Part model, mm, in its own coordinate system. A direction names the side the tool comes from. Give positions to 0.01 mm unless a question says otherwise; leave off trailing zeros. Write each loop counter-clockwise with the first axis right and the second up, starting at its lowest first coordinate (ties: lowest second). Pieces come first, ordered by that corner, then holes. Notation, with made-up numbers: M 27.5,27.25 L 54.5,27.25 A26 cw 54.5,62.25 Z; hole C -21.75,64 d1. An arc over 180 degrees is marked long. Answer as CSV lines item,"result". Start each with the question number.
1) Wall check: line 1 along X through (y, z) = (9.5, -1); line 2 along X through (y, z) = (20, 11.5); line 3 along Z through (x, y) = (13, 44). Give the ranges that are in metal, low to high. Write a range as from..to.
2) Slice it at A-A, the plane z = 0. Give the cut face in (x, y).
3) Slice it at D-D, the plane x = -25.5. Give the cut face in (y, z), plus the area to 3 significant figures.
4) Pin check, flat tips, straight feed: pin 1 Ø4 at (x, y) = (50, 12.5) entering from +Z; pin 2 Ø10 at (x, z) = (-51.5, -51) entering from +Y; pin 3 Ø2 at (y, z) = (23, -31.5) entering from -X; pin 4 Ø4 at (x, y) = (0, 38.1) entering from -Z. Stop position of each tip, or through.
5) Mould opens along Y. For faces 4 (the flat face through (-11.94, 27.94, -75.43)), 5 (the cylindrical face through (2.93, 36.88, -18)), 6 (the cylindrical face through (-45.395, 15.062, 62.776)) say: pulls with the +Y half, pulls with the -Y half, needs draft (parallel to the pull), parting line crosses it, or undercut.
6) Slice it at B-B, the plane x = 0. Give the number of separate pieces and of enclosed holes in the cut face, plus the area to 3 significant figures.
7) Tool access for faces 1 (the flat face through (-62, 27.94, -45)), 2 (the flat face through (-63.33, 41.41, -37.69)), 3 (the flat face through (37.69, 41.41, -63.33)): list every direction of +Z, -Z, +X, -X, +Y, -Y with a clear straight run to the whole face (end or side of a thin tool).
```python
from build123d import *

# Parameters (mm, degrees)
SKETCH2_R           = 76.2
BOSS_EXTRUDE1_DEPTH = 50.8
SKETCH3_R           = 71.12
SKETCH3_R_2         = 19.05
CUT_EXTRUDE1_DEPTH  = 44.45
SKETCH4_R           = 17.272
CUT_EXTRUDE2_DEPTH  = 120.1365603
CUT_EXTRUDE3_DEPTH  = 19.05
CIRPATTERN1_COUNT   = 8
SKETCH6_R           = 3.175
CUT_EXTRUDE4_DEPTH  = 25.4
WRAP1_START         = 2.54
WRAP1_DEPTH         = 25.4
CIRPATTERN2_COUNT   = 8


# Read off the part's stored shape, not the designer's step: Wrap1
with BuildPart() as part:
    # Sketch2 → Boss-Extrude1 (new body)
    with BuildSketch(Plane(origin=(0, 0, 0), x_dir=(1, 0, 0), z_dir=(0, 1, 0))):
        with Locations(Location((0, 0, 0), (0, 0, 270))):
            Circle(SKETCH2_R)
    extrude(amount=BOSS_EXTRUDE1_DEPTH)

    # Sketch3 → Cut-Extrude1 (cut)
    with BuildSketch(Plane(origin=(0, 50.8, 0), x_dir=(1, 0, 0), z_dir=(0, 1, 0))):
        with Locations(Location((0, 0, 0), (0, 0, 270))):
            Circle(SKETCH3_R)
        with Locations(Location((0, 0, 0), (0, 0, 270))):
            Circle(SKETCH3_R_2, mode=Mode.SUBTRACT)
    extrude(amount=-CUT_EXTRUDE1_DEPTH, mode=Mode.SUBTRACT)

    # Sketch4 → Cut-Extrude2 (cut, through all)
    with BuildSketch(Plane(origin=(0, 50.8, 0), x_dir=(1, 0, 0), z_dir=(0, 1, 0))):
        with Locations(Location((0, 0, 0), (0, 0, 270))):
            Circle(SKETCH4_R)
    extrude(amount=-CUT_EXTRUDE2_DEPTH, mode=Mode.SUBTRACT)

    # Sketch5 → Cut-Extrude3 (cut)
    with BuildSketch(Plane(origin=(0, 50.8, 0), x_dir=(1, 0, 0), z_dir=(0, 1, 0))):
        with BuildLine():
            Line((-44.991655358, 55.079990451), (-48.205345027, 59.014275484))
            ThreePointArc((-48.205345027, 59.014275484), (-57.719695429, 49.748133227), (-65.480674483, 38.970774553))
            Line((-65.480674483, 38.970774553), (-61.115296184, 36.372722916))
            ThreePointArc((-61.115296184, 36.372722916), (-53.871715734, 46.431591012), (-44.991655358, 55.079990451))
        make_face()
    cut_extrude3 = extrude(amount=-CUT_EXTRUDE3_DEPTH, mode=Mode.SUBTRACT)

    # CirPattern1: Cut-Extrude3 ×8 about axis
    cirpattern1_axis = Axis((0, 0, 0), (0, 1, 0))
    for i in range(1, CIRPATTERN1_COUNT):
        add(cut_extrude3.rotate(cirpattern1_axis, i * 360 / CIRPATTERN1_COUNT), mode=Mode.SUBTRACT)

    # Sketch6 → Cut-Extrude4 (cut, symmetric)
    with BuildSketch(Plane.XY):
        with Locations((0, 38.1)):
            Circle(SKETCH6_R)
    extrude(amount=CUT_EXTRUDE4_DEPTH, both=True, mode=Mode.SUBTRACT)

    # Wrap1 outline → Wrap1 (add)
    with BuildSketch(Plane(origin=(0, 0, 0), x_dir=(1, 0, 0), z_dir=(0, 1, 0)).offset(WRAP1_START)):
        with BuildLine():
            ThreePointArc((75.761080539, -16.182075751), (76.423312697, 12.691657751), (66.463869373, 39.801444294))
            Line((66.463869373, 39.801444294), (65.374297744, 39.148961601))
            ThreePointArc((65.374297744, 39.148961601), (75.170471505, 12.483597787), (74.519095612, -15.916795821))
            Line((74.519095612, -15.916795821), (75.761080539, -16.182075751))
        make_face()
    wrap1 = extrude(amount=WRAP1_DEPTH)

    # CirPattern2: Wrap1 ×8 about axis
    cirpattern2_axis = Axis((0, 0, 0), (0, 1, 0))
    for i in range(1, CIRPATTERN2_COUNT):
        add(wrap1.rotate(cirpattern2_axis, i * 360 / CIRPATTERN2_COUNT))


solid = part.part
```
Found:
1,line 1,"-77.46..-71.11, -19.02..-17.24, 17.24..19.02, 71.11..77.46"
1,line 2,"-76.61..-70.18, -15.19..-12.89, 12.89..15.19, 70.18..76.61"
1,line 3,"-75.08..-69.92, -13.92..-11.37, 11.37..13.92"
2,outline,"M -77.47,2.54 L -76.2,2.54 L -76.2,0 L -17.27,0 L -17.27,50.8 L -19.05,50.8 L -19.05,6.35 L -71.12,6.35 L -71.12,31.75 L -76.2,31.75 L -76.2,27.94 L -77.47,27.94 Z; M 17.27,0 L 76.2,0 L 76.2,2.54 L 77.47,2.54 L 77.47,27.94 L 76.2,27.94 L 76.2,31.75 L 71.12,31.75 L 71.12,6.35 L 19.05,6.35 L 19.05,50.8 L 17.27,50.8 Z"
3,outline,"M 0,-71.81 L 2.54,-71.81 L 2.54,-73.15 L 27.94,-73.15 L 27.94,-71.81 L 50.8,-71.81 L 50.8,-66.39 L 6.35,-66.39 L 6.35,66.39 L 50.8,66.39 L 50.8,71.81 L 27.94,71.81 L 27.94,73.15 L 2.54,73.15 L 2.54,71.81 L 0,71.81 Z"
3,area,"1,460 mm²"
4,pin 1,"z = 60.81"
4,pin 2,"y = 31.75"
4,pin 3,"x = -71.21"
4,pin 4,"through"
5,face 4,"pulls with the +Y half"
5,face 5,"undercut"
5,face 6,"needs draft"
6,separate pieces,"4"
6,enclosed holes,"0"
6,area,"1,210 mm²"
7,face 1,"-Z, -X, +Y"
7,face 2,"-Z, +Y"
7,face 3,"+X, +Y"
